Can you work these out from the drawing? Everything is in mm from the part's minimum corner. A direction names the side the tool comes from. Coordinates: 2 decimals unless noted, no trailing zeros. Loops run counter-clockwise (first coordinate to the right, second up) from the corner with the lowest first, then second, coordinate; pieces in that order, holes last.
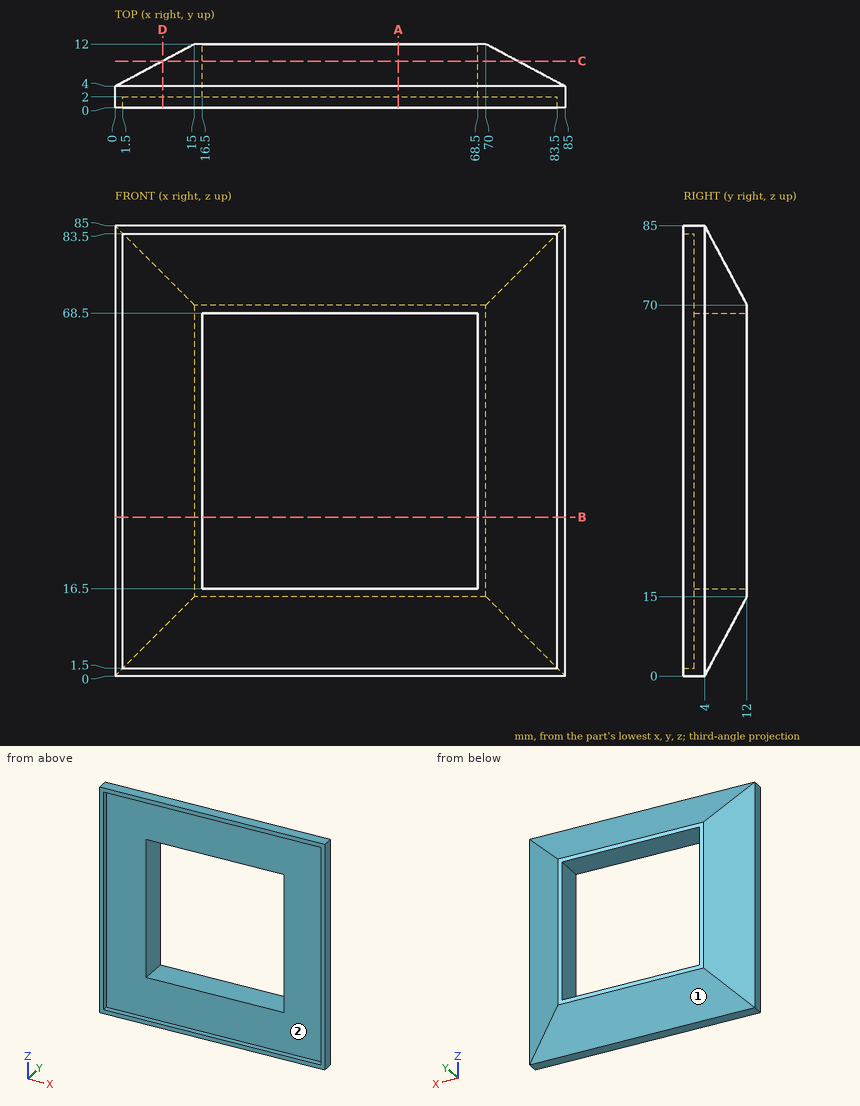
Item 1: Suppose I cut it at A-A, the plane x = 53.5. Please give me the cut outline in (y, z), plus the area to 3 significant figures.
Results are:
outline: (0, 0) - (4, 0) - (12, 15) - (12, 16.5) - (2, 16.5) - (2, 1.5) - (0, 1.5) - close; (0, 83.5) - (2, 83.5) - (2, 68.5) - (12, 68.5) - (12, 70) - (4, 85) - (0, 85) - close
area: 216 mm2
Item 2: I'm going to push flat-ended pins straight in: P1, Ø5, axis at x = 38, y = 8, coming from the -Z side; P2, Ø3, axis at x = 20.5, z = 16, coming from the -Y side; P3, Ø3, axis at x = 43, z = 9, coming from the +Y side. Where does each tip first touch, or does it pass through?
Results are:
P1: stops at z = 2.81
P2: stops at y = 2
P3: stops at y = 9.6
Item 3: On a 3-axis mill with a long thin cutter (end or side, diameter ignored), from which of +Z, -Z, +X, -X, +Y, -Y can I reach the whole of each face in a straight line? I mean the marked faces 1 and 2. Say none if no direction works.
Results are:
face 1: -Z, +X, -X, +Y
face 2: -Y
Item 4: I need wall thicknesses on line 1 along Z through (x, y) = (22.5, 1.5); line 2 along X through (y, z) = (7, 65) (3 decimals). Which ranges of each line are inside material? Lowest first, please.
Results are:
line 1: z = 0 to 1.5, 83.5 to 85
line 2: x = 5.625 to 16.5, 68.5 to 79.375
Item 5: Suppose I cut it at B-B, the plane z = 30. Please give me the cut outline in (x, y), plus the area to 3 significant figures.
Results are:
outline: (0, 0) - (1.5, 0) - (1.5, 2) - (16.5, 2) - (16.5, 12) - (15, 12) - (0, 4) - close; (68.5, 2) - (83.5, 2) - (83.5, 0) - (85, 0) - (85, 4) - (70, 12) - (68.5, 12) - close
area: 216 mm2
Item 6: Suppose I cut it at C-C, the plane y = 8.75. Please give me the cut outline in (x, z).
Results are:
outline: (8.91, 8.91) - (76.09, 8.91) - (76.09, 76.09) - (8.91, 76.09) - close; hole (16.5, 16.5) - (68.5, 16.5) - (68.5, 68.5) - (16.5, 68.5) - close
Item 7: Suppose I cut it at D-D, the plane x = 9. Please give me the cut outline in (y, z).
Results are:
outline: (0, 0) - (4, 0) - (8.8, 9) - (8.8, 76) - (4, 85) - (0, 85) - (0, 83.5) - (2, 83.5) - (2, 1.5) - (0, 1.5) - close
